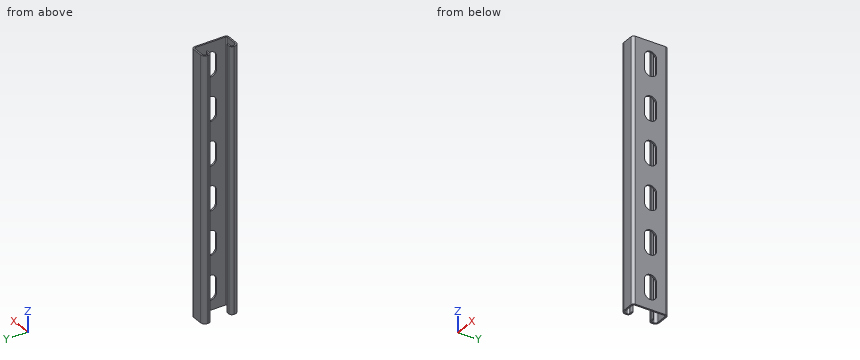
```python
from build123d import *

# Parameters (mm, degrees)
BOSS_EXTRUDE1_DEPTH = 304.8
CUT_EXTRUDE1_DEPTH  = 1.778
LPATTERN1_COUNT     = 6
LPATTERN1_PITCH     = 50.8


with BuildPart() as part:
    # Sketch1 → Boss-Extrude1 (new body)
    with BuildSketch(Plane.XY):
        with BuildLine():
            Line((-15.58925, 20.6375), (-3.46075, 20.6375))
            ThreePointArc((-3.46075, 20.6375), (-1.013630207, 19.623869793), (0, 17.17675))
            Line((0, 17.17675), (0, -17.17675))
            ThreePointArc((0, -17.17675), (-1.013630207, -19.623869793), (-3.46075, -20.6375))
            Line((-3.46075, -20.6375), (-15.58925, -20.6375))
            ThreePointArc((-15.58925, -20.6375), (-19.158901808, -19.158901808), (-20.6375, -15.58925))
            Line((-20.6375, -15.58925), (-20.6375, -14.57325))
            ThreePointArc((-20.6375, -14.57325), (-19.623869793, -12.126130207), (-17.17675, -11.1125))
            Line((-17.17675, -11.1125), (-14.3891, -11.1125))
            ThreePointArc((-14.3891, -11.1125), (-13.5001, -12.0015), (-14.3891, -12.8905))
            Line((-14.3891, -12.8905), (-17.17675, -12.8905))
            ThreePointArc((-17.17675, -12.8905), (-18.366633936, -13.383366064), (-18.8595, -14.57325))
            Line((-18.8595, -14.57325), (-18.8595, -15.58925))
            ThreePointArc((-18.8595, -15.58925), (-17.901665951, -17.901665951), (-15.58925, -18.8595))
            Line((-15.58925, -18.8595), (-3.46075, -18.8595))
            ThreePointArc((-3.46075, -18.8595), (-2.270866064, -18.366633936), (-1.778, -17.17675))
            Line((-1.778, -17.17675), (-1.778, 17.17675))
            ThreePointArc((-1.778, 17.17675), (-2.270866064, 18.366633936), (-3.46075, 18.8595))
            Line((-3.46075, 18.8595), (-15.58925, 18.8595))
            ThreePointArc((-15.58925, 18.8595), (-17.901665951, 17.901665951), (-18.8595, 15.58925))
            Line((-18.8595, 15.58925), (-18.8595, 14.57325))
            ThreePointArc((-18.8595, 14.57325), (-18.366633936, 13.383366064), (-17.17675, 12.8905))
            Line((-17.17675, 12.8905), (-14.3891, 12.8905))
            ThreePointArc((-14.3891, 12.8905), (-13.5001, 12.0015), (-14.3891, 11.1125))
            Line((-14.3891, 11.1125), (-17.17675, 11.1125))
            ThreePointArc((-17.17675, 11.1125), (-19.623869793, 12.126130207), (-20.6375, 14.57325))
            Line((-20.6375, 14.57325), (-20.6375, 15.58925))
            ThreePointArc((-20.6375, 15.58925), (-19.158901808, 19.158901808), (-15.58925, 20.6375))
        make_face()
    extrude(amount=-BOSS_EXTRUDE1_DEPTH)

    # Sketch2 → Cut-Extrude1 (cut)
    with BuildSketch(Plane(origin=(0, 0, 0), x_dir=(0, 0, -1), z_dir=(1, 0, 0))):
        with BuildLine():
            Line((18.25625, 7.14375), (32.54375, 7.14375))
            ThreePointArc((32.54375, 7.14375), (39.6875, 0), (32.54375, -7.14375))
            Line((32.54375, -7.14375), (18.25625, -7.14375))
            ThreePointArc((18.25625, -7.14375), (11.1125, 0), (18.25625, 7.14375))
        make_face()
    cut_extrude1 = extrude(amount=-CUT_EXTRUDE1_DEPTH, mode=Mode.SUBTRACT)

    # LPattern1: Cut-Extrude1 ×6
    with Locations(*[(0, 0, -i * LPATTERN1_PITCH) for i in range(1, LPATTERN1_COUNT)]):
        add(cut_extrude1, mode=Mode.SUBTRACT)


solid = part.part
```
The listing builds one solid part. Answer for the finished solid, in the listing's coordinates (mm). Give positions to 0.01 mm unless a question says otherwise; leave off trailing zeros. Loops run counter-clockwise (first coordinate to the right, second up) from the corner with the lowest first, then second, coordinate; pieces in that order, holes last. Notation, with made-up numbers: M 7.5,73.5 L 64.5,73.5 A11 ccw 64.5,87.5 Z; hole C 31.5,36.25 d10. An arc over 180 degrees is marked long. One line per item, written item: value.
Q1. A cutting plane is placed at B-B on z = -157. Determine the outline of the cut face in (x, y).
Working result:
outline: M -20.64,-15.59 A5.05 ccw -15.59,-20.64 L -3.46,-20.64 A3.46 ccw 0,-17.18 L 0,17.18 A3.46 ccw -3.46,20.64 L -15.59,20.64 A5.05 ccw -20.64,15.59 L -20.64,14.57 A3.46 ccw -17.18,11.11 L -14.39,11.11 A0.89 ccw -14.39,12.89 L -17.18,12.89 A1.68 cw -18.86,14.57 L -18.86,15.59 A3.27 cw -15.59,18.86 L -3.46,18.86 A1.68 cw -1.78,17.18 L -1.78,-17.18 A1.68 cw -3.46,-18.86 L -15.59,-18.86 A3.27 cw -18.86,-15.59 L -18.86,-14.57 A1.68 cw -17.18,-12.89 L -14.39,-12.89 A0.89 ccw -14.39,-11.11 L -17.18,-11.11 A3.46 ccw -20.64,-14.57 Z
Q2. Find the intervals of material crossed by line 1 (Y direction, x = -16, z = -166); line 2 (Y direction, x = -8.5, z = -191); line 3 (Y direction, x = -15.5, z = -183), in increasing order. Write a range as from..to.
Working result:
line 1: y = -20.62..-18.83, -12.89..-11.11, 11.11..12.89, 18.83..20.62
line 2: y = -20.64..-18.86, 18.86..20.64
line 3: y = -20.64..-18.86, -12.89..-11.11, 11.11..12.89, 18.86..20.64
Q3. A cutting plane is placed at C-C on x = -7.5. Determine the outline of the cut face in (y, z), then the cut area to 3 significant figures.
Working result:
outline: M -20.64,-304.8 L -18.86,-304.8 L -18.86,0 L -20.64,0 Z; M 18.86,-304.8 L 20.64,-304.8 L 20.64,0 L 18.86,0 Z
area: 1,080 mm^2
Q4. A cutting plane is placed at A-A on y = 0. Determine the outline of the cut face in (x, z).
Working result:
outline: M -1.78,-304.8 L 0,-304.8 L 0,-293.69 L -1.78,-293.69 Z; M -1.78,-265.11 L 0,-265.11 L 0,-242.89 L -1.78,-242.89 Z; M -1.78,-214.31 L 0,-214.31 L 0,-192.09 L -1.78,-192.09 Z; M -1.78,-163.51 L 0,-163.51 L 0,-141.29 L -1.78,-141.29 Z; M -1.78,-112.71 L 0,-112.71 L 0,-90.49 L -1.78,-90.49 Z; M -1.78,-61.91 L 0,-61.91 L 0,-39.69 L -1.78,-39.69 Z; M -1.78,-11.11 L 0,-11.11 L 0,0 L -1.78,0 Z
Q5. Flat-ended cylindrical pins translate along their axes: P1, Ø1.4, axis at x = -1.5, z = -281, coming from the -Y side; P2, Ø2, axis at x = -0.5, z = -74, coming from the -Y side; P3, Ø1.4, axis at x = -1, z = -127.5, coming from the -Y side. Find the tip coordinate at first contact, or state that the pin passes through.
Working result:
P1: stops at y = -20.4
P2: stops at y = -20.03
P3: stops at y = -20.16
